Geometry: see drawing. Coordinates: mm, zero at the bounding-box minimum. Coordinates: 2 decimals unless noted, no trailing zeros. Order: outer loops, then holes, each group sorted by start corner. A loop starts at its lowest first (then second) coordinate and runs counter-clockwise, first axis right, second up.
Item 1: Mould query, pull axis X, two halves, no side actions, for the marked faces 1, 2 and 3. Classes: released by +X, released by -X, zero draft, split by the parting line, or undercut.
Item 2: Section B-B on z = 5.5. Return the cut outline in (x, y).
Item 3: Section C-C on x = 19.5. Return the cut outline in (y, z).
Item 4: Ray query, line 1 (X direction, y = 19, z = 32); line 2 (X direction, y = 33, z = 23.5) (1 decimal); line 3 (Z direction, x = 13, y = 19.5) (1 decimal). Return the intervals inside material, ascending.
Item 5: Contact query for flat-ended pins moving along their axis: P1, Ø1.5, axis at y = 36, z = 21, coming from the +X side; P2, Ø6, axis at y = 44.5, z = 8, coming from the +X side; P3, Ø4, axis at y = 8.5, z = 23.5, coming from the -X side. Output: stop coordinate, or through.
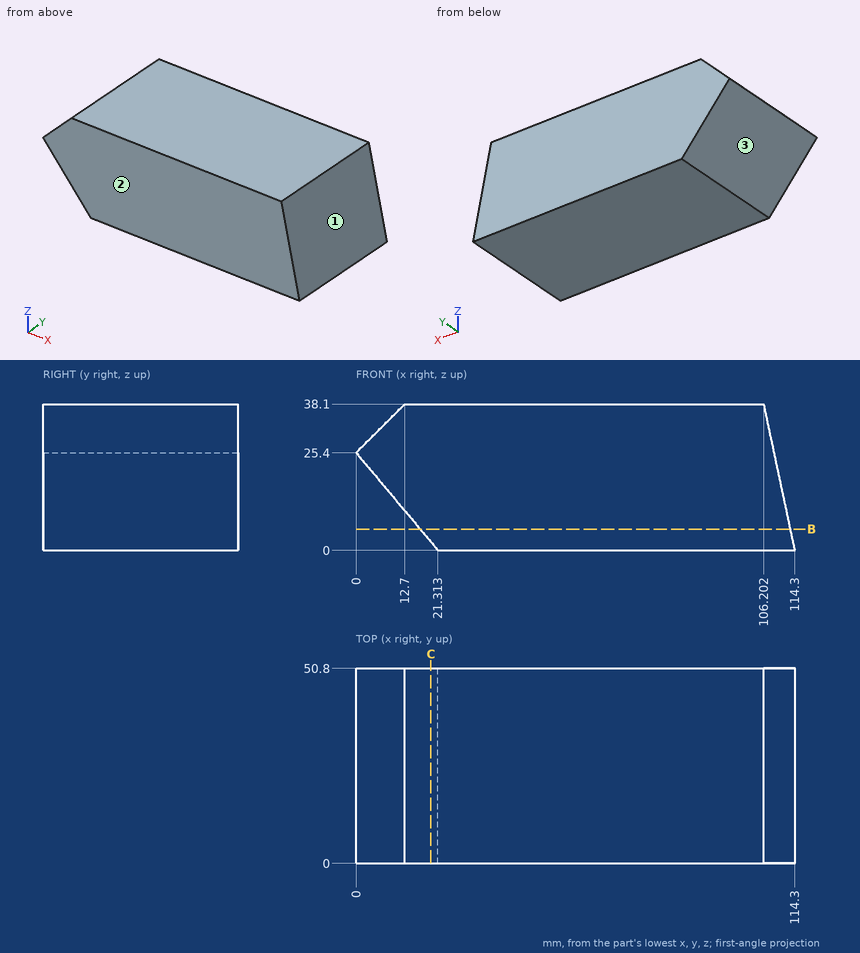
Answer list:
1. face 1: released by +X
1. face 2: zero draft
1. face 3: released by -X
2. outline: (16.7, 0) - (113.13, 0) - (113.13, 50.8) - (16.7, 50.8) - close
3. outline: (0, 2.16) - (50.8, 2.16) - (50.8, 38.1) - (0, 38.1) - close
4. line 1: x = 6.6 to 107.5
4. line 2: x = 1.6 to 109.3
4. line 3: z = 9.9 to 38.1
5. P1: stops at x = 110
5. P2: stops at x = 113.24
5. P3: stops at x = 0
